```python
from build123d import *

# Parameters (mm, degrees)
EXTRUDE_1_DEPTH     = 7
CUT_EXTRUDE_START   = -5.1
CUT_EXTRUDE_1_DEPTH = 5.1
CUT_EXTRUDE_START_2 = -2.5
CUT_EXTRUDE_2_DEPTH = 2.5


with BuildPart() as part:
    # Эскиз1 → Бобышка-Вытянуть1 (new body)
    with BuildSketch(Plane.XY):
        with BuildLine():
            Line((-17.15601973, -7.7), (-30.620254734, -1.35))
            ThreePointArc((-30.620254734, -1.35), (-30.65, 0), (-30.620254734, 1.35))
            Line((-30.620254734, 1.35), (-17.15601973, 7.7))
            Line((-17.15601973, 7.7), (-4.15601973, 7.7))
            ThreePointArc((-4.15601973, 7.7), (-8.75, 0), (-4.15601973, -7.7))
            Line((-4.15601973, -7.7), (-17.15601973, -7.7))
        make_face()
    extrude(amount=EXTRUDE_1_DEPTH)

    # Эскиз2 → Вырез-Вытянуть1 (cut)
    with BuildSketch(Plane.XY.offset(7).offset(CUT_EXTRUDE_START)):
        with BuildLine():
            Line((-4.15601973, 7.7), (-17, 7.7))
            Line((-17, 7.7), (-17, -7.7))
            Line((-17, -7.7), (-4.15601973, -7.7))
            ThreePointArc((-4.15601973, -7.7), (-8.75, 0), (-4.15601973, 7.7))
        make_face()
    extrude(amount=CUT_EXTRUDE_1_DEPTH, mode=Mode.SUBTRACT)

    # Эскиз2<5> → Вырез-Вытянуть2 (cut)
    with BuildSketch(Plane.XY.offset(7).offset(CUT_EXTRUDE_START_2)):
        with BuildLine():
            Line((-17, -7.7), (-17, 7.7))
            Line((-17, 7.7), (-17.15601973, 7.7))
            Line((-17.15601973, 7.7), (-30.620254734, 1.35))
            ThreePointArc((-30.620254734, 1.35), (-30.65, 0), (-30.620254734, -1.35))
            Line((-30.620254734, -1.35), (-17.15601973, -7.7))
            Line((-17.15601973, -7.7), (-17, -7.7))
        make_face()
    extrude(amount=CUT_EXTRUDE_2_DEPTH, mode=Mode.SUBTRACT)


solid = part.part
```
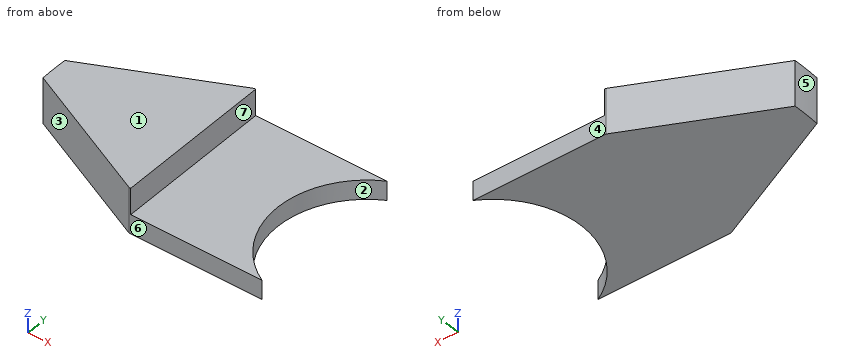
Geometry: final body of the model. Coordinates: model frame, mm. Face numbers are marked on the shaded views. A direction names the side the tool comes from. Give positions to 0.01 mm unless a question says otherwise; leave off trailing zeros. Order: outer loops, then holes, each group sorted by start corner. A loop starts at its lowest first (then second) coordinate and runs counter-clockwise, first axis right, second up. Notation, with made-up numbers: (1, -19.5) -> (39, -19.5) arc R18 ccw to (39, 9.5) -> close; hole circle Ø10 at (18, 4.5). An arc over 180 degrees is marked (long way). Write each question's results on one line, items separated by ' | '. Start each with the question number.
1) Section B-B (y = -5.75). Return loops of the section in (x, z).
2) Set-up query: the marked faces 5, 6 and 7. Return all of +Z, -Z, +X, -X, +Y, -Y with unobstructed straight access to the full face (end or side cutting, diameter ignored); none if empty.
3) Line query: line 1 (Y direction, x = -7, z = 1.25); line 2 (Z direction, x = -12.5, y = 3.5); line 3 (Y direction, x = -27.5, z = 1). Output: solid intervals per line, ascending. Write a range as from..to.
4) Section C-C (x = -10.5). Return loops of the section in (y, z), then the cut area to 3 significant figures.
5) Section A-A (z = 0.7). Return loops of the section in (x, y).
6) Draft query along Y for the marked faces 1, 2, 3 and 4. Return one class per face: pulls with the +Y half, pulls with the -Y half, needs draft (parallel to the pull), parting line crosses it, or undercut.
7) First-contact query: pin 1 (1 mm diameter, centred on y = -4, z = 1, fed in from +X); pin 2 (1.5 mm diameter, centred on x = -24, y = -5.5, fed in from +Z); pin 3 (0.8 mm diameter, centred on y = -3, z = 3.5, fed in from +X). Flat tips, straight axial feed; report the tip coordinate or a pass-through.
8) Section D-D (x = -19). Return loops of the section in (y, z), then the cut area to 3 significant figures.
Calculated:
1) outline: (-21.29, 0) -> (-6.6, 0) -> (-6.6, 1.9) -> (-17, 1.9) -> (-17, 4.5) -> (-21.29, 4.5) -> close
2) face 5: +Z, -Z, -X | face 6: +Z, -Z, +X, -X, -Y | face 7: +Z, +X, +Y, -Y
3) line 1: -7.7..-5.25, 5.25..7.7 | line 2: 0..1.9 | line 3: -2.82..2.82
4) outline: (-7.7, 0) -> (7.7, 0) -> (7.7, 1.9) -> (-7.7, 1.9) -> close | area: 29.3 mm2
5) outline: (-30.62, -1.35) -> (-17.16, -7.7) -> (-4.16, -7.7) arc R8.75 cw to (-4.16, 7.7) -> (-17.16, 7.7) -> (-30.62, 1.35) arc R30.65 ccw to start
6) face 1: needs draft | face 2: undercut | face 3: pulls with the -Y half | face 4: pulls with the +Y half
7) pin 1: x = -7.5 | pin 2: through | pin 3: x = -17
8) outline: (-6.83, 0) -> (6.83, 0) -> (6.83, 4.5) -> (-6.83, 4.5) -> close | area: 61.5 mm2
